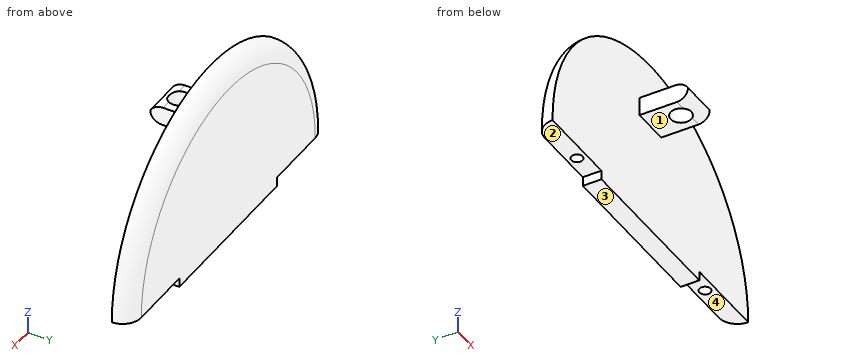
from build123d import *

# Parameters (mm, degrees)
CUT_EXTRUDE1_DEPTH           = 5
CUT_EXTRUDE3_DEPTH           = 45
SKETCH8_R                    = 43
CUT_EXTRUDE4_DEPTH           = 32
SKETCH9_R                    = 32
SKETCH9_R_2                  = 24.5
CUT_EXTRUDE5_DEPTH           = 14
SKETCH10_R                   = 26
CUT_EXTRUDE6_DEPTH           = 14
FILLET1_R                    = 7
FILLET2_R                    = 7
SKETCH12_W                   = 6.590120242
SKETCH12_H                   = 30.5
CUT_REVOLVE1_ANGLE           = 60
CUT_REVOLVE1_OTHER_WAY_ANGLE = 60
CUT_EXTRUDE12_DEPTH          = 5
SKETCH18_W                   = 13
SKETCH18_H                   = 8
CUT_EXTRUDE13_DEPTH          = 5
INTERSECT1_OUTLINE_R         = 45
INTERSECT1_DEPTH             = 79
SKETCH20_W                   = 10
SKETCH20_H                   = 5
BOSS_EXTRUDE1_DEPTH          = 13
BOSS_EXTRUDE3_DEPTH          = 5
SKETCH19_R                   = 1.5
CUT_EXTRUDE14_DEPTH          = 20
SKETCH23_W                   = 25
SKETCH23_H                   = 7
CUT_EXTRUDE15_DEPTH          = 7
SKETCH24_W                   = 45
SKETCH24_H                   = 2.5
CUT_EXTRUDE16_DEPTH          = 5
SKETCH25_R                   = 2.75
CUT_EXTRUDE17_DEPTH          = 5
FILLET4_R                    = 3
FILLET6_R                    = 4


with BuildPart() as part:
    # Sketch1 → Revolve1 (revolve)
    with BuildSketch(Plane.XY, mode=Mode.PRIVATE) as revolve1_sk:
        with BuildLine():
            Line((22.5, 0), (32, 0))
            ThreePointArc((32, 0), (33.414213562, 0.585786438), (34, 2))
            Line((34, 2), (34, 18))
            Line((34, 18), (43, 18))
            ThreePointArc((43, 18), (44.414213562, 18.585786438), (45, 20))
            Line((45, 20), (45, 79))
            ThreePointArc((45, 79), (43.535533906, 82.535533906), (40, 84))
            Line((40, 84), (0, 84))
            Line((0, 84), (0, 18))
            Line((0, 18), (22.5, 18))
            Line((22.5, 18), (22.5, 0))
        make_face()
    revolve(revolve1_sk.sketch.rotate(Axis((0, 2, 0), (0, 1, 0)), 90), axis=Axis((0, 2, 0), (0, 1, 0)))

    # Sketch5 → Cut-Extrude1 (cut)
    with BuildSketch(Plane(origin=(0, 84, 0), x_dir=(1, 0, 0), z_dir=(0, 1, 0))):
        with BuildLine():
            Line((-45, 0), (-40, 0))
            Line((-40, 0), (40, 0))
            Line((40, 0), (45, 0))
            ThreePointArc((45, 0), (0, 45), (-45, 0))
        make_face()
    extrude(amount=-CUT_EXTRUDE1_DEPTH, mode=Mode.SUBTRACT)

    # Sketch7 → Cut-Extrude3 (cut)
    with BuildSketch(Plane.XZ.offset(-18)):
        with BuildLine():
            Line((-21, 0), (21, 0))
            ThreePointArc((21, 0), (0, -21), (-21, 0))
        make_face()
    extrude(amount=-CUT_EXTRUDE3_DEPTH, mode=Mode.SUBTRACT)

    # Sketch8 → Cut-Extrude4 (cut)
    with BuildSketch(Plane(origin=(0, 76.5, 0), x_dir=(1, 0, 0), z_dir=(0, 1, 0))):
        with Locations(Location((0, 0, 0), (0, 0, 270))):
            Circle(SKETCH8_R)
        with BuildLine():
            Line((22.912878475, -2), (-22.912878475, -2))
            ThreePointArc((-22.912878475, -2), (0, 23), (22.912878475, -2))
        make_face(mode=Mode.SUBTRACT)
    extrude(amount=-CUT_EXTRUDE4_DEPTH, mode=Mode.SUBTRACT)

    # Sketch9 → Cut-Extrude5 (cut)
    with BuildSketch(Plane(origin=(0, 2, 0), x_dir=(-1, 0, 0), z_dir=(0, -1, 0))):
        with Locations(Location((0, 0, 0), (0, 0, 90))):
            Circle(SKETCH9_R)
        with Locations(Location((0, 0, 0), (0, 0, 90))):
            Circle(SKETCH9_R_2, mode=Mode.SUBTRACT)
    extrude(amount=-CUT_EXTRUDE5_DEPTH, mode=Mode.SUBTRACT)

    # Sketch10 → Cut-Extrude6 (cut)
    with BuildSketch(Plane(origin=(0, 2, 0), x_dir=(-1, 0, 0), z_dir=(0, -1, 0))):
        Circle(SKETCH10_R)
    extrude(amount=-CUT_EXTRUDE6_DEPTH, mode=Mode.SUBTRACT)

    # Fillet1
    fillet1_edges = [part.edges().sort_by_distance(p)[0] for p in [
        (21, 40.5, 0),
        (-21, 40.5, 0),
    ]]
    fillet(fillet1_edges, radius=FILLET1_R)

    # Fillet2
    fillet2_edges = [part.edges().sort_by_distance(p)[0] for p in [
        (-22.912878475, 60.5, 2),
        (22.912878475, 60.5, 2),
    ]]
    fillet(fillet2_edges, radius=FILLET2_R)

    # Sketch12 → Cut-Revolve1 (revolve, cut)
    with BuildSketch(Plane(origin=(0, 0, 0), x_dir=(0, 0, -1), z_dir=(1, 0, 0))):
        with Locations((-40.662298382, 61.25)):
            Rectangle(SKETCH12_W, SKETCH12_H)
    revolve(axis=Axis((0, 99.14944168, 0), (0, 1, 0)), revolution_arc=CUT_REVOLVE1_ANGLE, mode=Mode.SUBTRACT)

    # Sketch12 → Cut-Revolve1 other way (revolve, cut)
    with BuildSketch(Plane(origin=(0, 0, 0), x_dir=(0, 0, -1), z_dir=(1, 0, 0))):
        with Locations((-40.662298382, 61.25)):
            Rectangle(SKETCH12_W, SKETCH12_H)
    revolve(axis=Axis((0, 99.14944168, 0), (0, -1, 0)), revolution_arc=CUT_REVOLVE1_OTHER_WAY_ANGLE, mode=Mode.SUBTRACT)

    # Sketch15 → Cut-Extrude12 (cut)
    with BuildSketch(Plane(origin=(0, 44.5, 0), x_dir=(1, 0, 0), z_dir=(0, 1, 0))):
        with BuildLine():
            Line((-28.124355653, -3.514579578), (-26.124355653, -3.514579578))
            ThreePointArc((-26.124355653, -3.514579578), (-24.710142091, -2.928793141), (-24.124355653, -1.514579578))
            Line((-24.124355653, -1.514579578), (-24.124355653, 8.485420422))
            ThreePointArc((-24.124355653, 8.485420422), (-24.710142091, 9.899633984), (-26.124355653, 10.485420422))
            Line((-26.124355653, 10.485420422), (-28.124355653, 10.485420422))
            ThreePointArc((-28.124355653, 10.485420422), (-29.538569215, 9.899633984), (-30.124355653, 8.485420422))
            Line((-30.124355653, 8.485420422), (-30.124355653, -1.514579578))
            ThreePointArc((-30.124355653, -1.514579578), (-29.538569215, -2.928793141), (-28.124355653, -3.514579578))
        make_face()
    extrude(amount=-CUT_EXTRUDE12_DEPTH, mode=Mode.SUBTRACT)

    # Sketch18 → Cut-Extrude13 (cut)
    with BuildSketch(Plane(origin=(0, 79, 0), x_dir=(1, 0, 0), z_dir=(0, 1, 0))):
        with Locations((0.796512215, 32.951769165)):
            Rectangle(SKETCH18_W, SKETCH18_H)
    extrude(amount=-CUT_EXTRUDE13_DEPTH, mode=Mode.SUBTRACT)

    # Intersect1: read off the stored shape, not the designer's step
    # Intersect1 outline → Intersect1 (cut)
    with BuildSketch(Plane(origin=(0, 0, 0), x_dir=(1, 0, 0), z_dir=(0, 1, 0))):
        Circle(INTERSECT1_OUTLINE_R)
    extrude(amount=INTERSECT1_DEPTH, mode=Mode.SUBTRACT)

    # Sketch20 → Boss-Extrude1 (add)
    with BuildSketch(Plane.XZ.offset(-79)):
        with Locations((0, 30)):
            Rectangle(SKETCH20_W, SKETCH20_H)
    extrude(amount=BOSS_EXTRUDE1_DEPTH)

    # Sketch22 → Boss-Extrude3 (add)
    with BuildSketch(Plane(origin=(0, 0, 0), x_dir=(-1, 0, 0), z_dir=(0, 0, -1))):
        with BuildLine():
            Line((40, 84), (-40, 84))
            ThreePointArc((-40, 84), (-43.535533906, 82.535533906), (-45, 79))
            Line((-45, 79), (45, 79))
            ThreePointArc((45, 79), (43.535533906, 82.535533906), (40, 84))
        make_face()
    extrude(amount=BOSS_EXTRUDE3_DEPTH)

    # Sketch19 → Cut-Extrude14 (cut)
    with BuildSketch(Plane(origin=(0, 0, 0), x_dir=(-1, 0, 0), z_dir=(0, 0, -1))):
        with Locations((0, 81.5)):
            Circle(SKETCH19_R)
        with Locations((-29.45, 81.5)):
            Circle(SKETCH19_R)
        with Locations((29.45, 81.5)):
            Circle(SKETCH19_R)
    extrude(amount=-CUT_EXTRUDE14_DEPTH, mode=Mode.SUBTRACT)

    # Sketch23 → Cut-Extrude15 (cut)
    with BuildSketch(Plane(origin=(0, 84, 0), x_dir=(1, 0, 0), z_dir=(0, 1, 0))):
        with Locations((-35, 3.5)):
            Rectangle(SKETCH23_W, SKETCH23_H)
        with Locations((35, 3.5)):
            Rectangle(SKETCH23_W, SKETCH23_H)
    extrude(amount=-CUT_EXTRUDE15_DEPTH, mode=Mode.SUBTRACT)

    # Sketch24 → Cut-Extrude16 (cut)
    with BuildSketch(Plane(origin=(0, 84, 0), x_dir=(1, 0, 0), z_dir=(0, 1, 0))):
        with Locations((0, 3.75)):
            Rectangle(SKETCH24_W, SKETCH24_H)
    extrude(amount=-CUT_EXTRUDE16_DEPTH, mode=Mode.SUBTRACT)

    # Sketch25 → Cut-Extrude17 (cut)
    with BuildSketch(Plane(origin=(0, 0, 27.5), x_dir=(-1, 0, 0), z_dir=(0, 0, -1))):
        with Locations((0, 70.8)):
            Circle(SKETCH25_R)
    extrude(amount=-CUT_EXTRUDE17_DEPTH, mode=Mode.SUBTRACT)

    # Fillet4
    # the kernel refuses this fillet: 3 mm, written as the material it takes off along each edge
    with BuildSketch(Plane(origin=(12.5, 66, 27.5), x_dir=(0, 1, 0), z_dir=(-1, 0, 0))) as fillet4_piece_1:
        with BuildLine():
            CenterArc((FILLET4_R, -FILLET4_R), FILLET4_R, 90, 90)
            Line((0, -FILLET4_R), (0, 0))
            Line((0, 0), (FILLET4_R, 0))
        make_face()
    extrude(amount=25, mode=Mode.SUBTRACT)

    # Fillet6
    # the kernel refuses this fillet: 4 mm, written as the material it takes off along each edge
    with BuildSketch(Plane(origin=(-13.660254038, 66, 32.5), x_dir=(0, 1, 0), z_dir=(1, 0, 0))) as fillet6_piece_1:
        with BuildLine():
            CenterArc((3.464101615, -4), FILLET6_R, 90, 60)
            Line((0, -2), (0, 0))
            Line((0, 0), (3.464101615, 0))
        make_face()
    extrude(amount=27.320508076, mode=Mode.SUBTRACT)


solid = part.part
Geometry check sheet. Reference: the model listing, model coordinates, mm. Face numbers are marked on the shaded views. A direction names the side the tool comes from. Coordinates: 2 decimals unless noted, no trailing zeros. Loops run counter-clockwise (first coordinate to the right, second up) from the corner with the lowest first, then second, coordinate; pieces in that order, holes last. Notation, with made-up numbers: (87, 27.25) - (141, 27.25) arc R29 cw to (141, 47.25) - close; hole circle Ø4 at (80.25, 53.5). An arc over 180 degrees is marked (long way). Use one line per item in the form item = value. Start each with the question number.
Item 1: Section check C-C, the plane y = 81.5. Enter the section's corners in (x, z).
Item 2: Section check B-B, the plane x = 0. Enter the section's corners in (y, z), and give its area (3 significant figures).
Item 3: Thickness scan on probe 1 along X at (y, z) = (81.5, 13.25); probe 2 along X at (y, z) = (81.5, 9.75); probe 3 along Y at (x, z) = (0, 5). Record the ranges inside material, lowest first.
Item 4: Section check A-A, the plane y = 70.8. Enter the section's corners in (x, z), and give its area (3 significant figures).
Item 5: Tool access check on the marked faces 1, 2, 3 and 4. Record the directions out of +Z, -Z, +X, -X, +Y, -Y that give a thin tool (end or side, any length) a straight path to the whole face; none if there is none.
Item 6: Section check D-D, the plane z = 16.5. Give the number of separate pieces and of enclosed holes in the cut face, and give its area (3 significant figures).
Item 7: Gauge pin test, flat ends, axial feed: pin 1 (1.5 mm diameter, centred on x = 33.5, y = 82, fed in from -Z); pin 2 (4 mm diameter, centred on x = 34, z = 25.5, fed in from +Y); pin 3 (0.8 mm diameter, centred on y = 82.5, z = -1, fed in from -X); pin 4 (4.5 mm diameter, centred on x = 0, y = 70.8, fed in from +Z). Record the tip position at first contact, or that the pin passes through.
Computed:
q1.outline = (-44.33, 0) - (-30.95, 0) - (-30.95, 20) - (-27.95, 20) - (-27.95, 0) - (-22.5, 0) - (-22.5, -2.5) - (22.5, -2.5) - (22.5, 0) - (27.95, 0) - (27.95, 20) - (30.95, 20) - (30.95, 0) - (44.33, 0) arc R44.33 ccw to start; hole (-1.5, 0) - (1.5, 0) - (1.5, 20) - (-1.5, 20) - close
q2.outline = (66, 30.5) arc R3 ccw to (68.05, 27.65) - (68.05, 32.24) arc R4 ccw to start; (73.55, 27.5) - (79, 27.5) - (79, -2.5) - (84, -2.5) - (84, 40) arc R5 ccw to (79, 45) - (79, 32.5) - (73.55, 32.5) - close; hole (80, 0) - (83, 0) - (83, 20) - (80, 20) - close
q2.area = 206 mm2
q3.probe_1 = -42.3 to -30.95, -27.95 to -1.5, 1.5 to 27.95, 30.95 to 42.3
q3.probe_2 = -43.24 to -30.95, -27.95 to -1.5, 1.5 to 27.95, 30.95 to 43.24
q3.probe_3 = 79 to 80, 83 to 84
q4.outline = (-5, 27.5) - (-2.75, 27.5) - (-2.75, 32.5) - (-5, 32.5) - close; (2.75, 27.5) - (5, 27.5) - (5, 32.5) - (2.75, 32.5) - close
q4.area = 22.5 mm2
q5.face_1 = -Z, +X, -X, -Y
q5.face_2 = -Z, -X, +Y, -Y
q5.face_3 = -Z, +X, -X, +Y, -Y
q5.face_4 = -Z, +X, +Y, -Y
q6.separate_pieces = 1
q6.enclosed_holes = 3
q6.area = 386 mm2
q7.pin_1 = 0
q7.pin_2 = 83.97
q7.pin_3 = -22.5
q7.pin_4 = through
